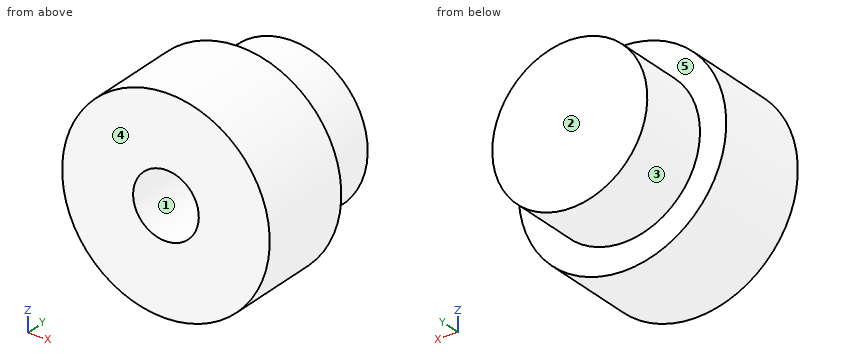
from build123d import *

# Parameters (mm, degrees)
SKETCH2_R          = 2.5
CUT_EXTRUDE1_DEPTH = 10


with BuildPart() as part:
    # Sketch1 → Revolve1 (revolve)
    with BuildSketch(Plane.XY, mode=Mode.PRIVATE) as revolve1_sk:
        Polygon((0, 0), (7.9, 0), (7.9, 7.5), (5.9, 7.5), (5.9, 13.022374429), (0, 13.022374429), align=None)
    revolve(revolve1_sk.sketch.rotate(Axis((0, 13.022374429, 0), (0, -1, 0)), 90), axis=Axis((0, 13.022374429, 0), (0, -1, 0)))

    # Sketch2 → Cut-Extrude1 (cut)
    with BuildSketch(Plane.XZ):
        with Locations(Location((0, 0, 0), (0, 0, 270))):
            Circle(SKETCH2_R)
    extrude(amount=-CUT_EXTRUDE1_DEPTH, mode=Mode.SUBTRACT)


solid = part.part
The model under review builds one solid part; all positions refer to its coordinate system, in mm. Face numbers are marked on the shaded views. A direction names the side the tool comes from. Round coordinates to 2 decimals unless told otherwise and drop trailing zeros. Order: outer loops, then holes, each group sorted by start corner. A loop starts at its lowest first (then second) coordinate and runs counter-clockwise, first axis right, second up. Notation, with made-up numbers: (-25, -4.5) -> (4, -4.5) arc R22 cw to (4, 11.5) -> close; hole circle Ø8 at (73, -5.75). An arc over 180 degrees is marked (long way). Write item = value, one per line. Start each with the question number.
Item 1: Clearance check with flat-ended pins moving along their axes: pin 1 Ø2 at (y, z) = (11, -5) entering from +X; pin 2 Ø1.5 at (y, z) = (1.5, 2.5) entering from -X; pin 3 Ø6 at (x, y) = (5.5, 8.5) entering from -Z. State where each tip first meets the part, or that it passes through.
Item 2: Consider section B-B on x = 0. Write out the cut boundary in (y, z), plus the area to 3 significant figures.
Item 3: Mouldability with a two-part tool opening along X and no side actions: class the marked faces 1, 2 and 3 as released by +X, released by -X, zero draft, split by the parting line, or undercut.
Item 4: Consider section D-D on z = -3.25. Write out the cut boundary in (x, y), plus the area to 3 significant figures.
Item 5: Consider section C-C on y = 9.75. Write out the cut boundary in (x, z), plus the area to 3 significant figures.
Item 6: For the marked faces 4 and 5, list the 3-axis set-ups (+Z, -Z, +X, -X, +Y, -Y) from which the entire face can be reached by the end or side of a thin tool; tool diameter is ignored.
Item 7: For line 1 along X through (y, z) = (2.5, 0); line 2 along Y through (x, z) = (1, -0.25); line 3 along Y through (x, z) = (6.75, -1), list the stretches that pass through material, from the lowest coordinate up.
Item 8: Consider section A-A on z = 0. Write out the cut boundary in (x, y).
Conclusion:
q1.pin_1 = 4.34
q1.pin_2 = -7.7
q1.pin_3 = -7.43
q2.outline = (0, -7.9) -> (7.5, -7.9) -> (7.5, -5.9) -> (13.02, -5.9) -> (13.02, 5.9) -> (7.5, 5.9) -> (7.5, 7.9) -> (0, 7.9) -> (0, 2.5) -> (10, 2.5) -> (10, -2.5) -> (0, -2.5) -> close
q2.area = 134 mm2
q3.face_1 = undercut
q3.face_2 = zero draft
q3.face_3 = split by the parting line
q4.outline = (-7.2, 0) -> (7.2, 0) -> (7.2, 7.5) -> (4.92, 7.5) -> (4.92, 13.02) -> (-4.92, 13.02) -> (-4.92, 7.5) -> (-7.2, 7.5) -> close
q4.area = 162 mm2
q5.outline = circle Ø11.8 at (0, 0); hole circle Ø5 at (0, 0)
q5.area = 89.7 mm2
q6.face_4 = +Z, -Z, +X, -X, -Y
q6.face_5 = +Y
q7.line_1 = -7.9 to -2.5, 2.5 to 7.9
q7.line_2 = 10 to 13.02
q7.line_3 = 0 to 7.5
q8.outline = (-7.9, 0) -> (-2.5, 0) -> (-2.5, 10) -> (2.5, 10) -> (2.5, 0) -> (7.9, 0) -> (7.9, 7.5) -> (5.9, 7.5) -> (5.9, 13.02) -> (-5.9, 13.02) -> (-5.9, 7.5) -> (-7.9, 7.5) -> close
